Verification items for this drawing (mm, ordinates from the low corner). A direction names the side the tool comes from. Give positions to 0.01 mm unless a question says otherwise; leave off trailing zeros. Write each loop counter-clockwise with the first axis right and the second up, starting at its lowest first coordinate (ties: lowest second). Pieces come first, ordered by that corner, then holes. Notation, with made-up numbers: (-5.75, -5) -> (30.25, -5) arc R15 cw to (30.25, 4) -> close; hole circle Ø9 at (82.5, 22.25). An arc over 180 degrees is marked (long way). Use one line per item in the form item = value. Start each with the question number.
(1) Set-up check for the marked faces 4, 5 and 6: record each of +Z, -Z, +X, -X, +Y, -Y from which the full face is reachable in a straight line by a thin tool's end or side.
(2) Section check B-B, the plane z = 7. Record the cut outline in (x, y).
(3) Release check for a two-part mould opening along Y. For the marked faces 1, 2 and 3 record: pulls with the +Y half, pulls with the -Y half, needs draft (parallel to the pull), parting line crosses it, or undercut.
(4) Depth check by flat-ended pin: pin 1 Ø6 at (x, z) = (14.5, 14.5) entering from -Y; pin 2 Ø4 at (x, y) = (2.5, 229) entering from +Z; pin 3 Ø16.5 at (y, z) = (98.5, 48) entering from -X; pin 4 Ø8 at (x, y) = (36.5, 191.5) entering from -Z. Enter the tip coordinate at first touch or a pass-through.
(5) Section check A-A, the plane x = 55. Record the cut outline in (y, z).
(6) Section check D-D, the plane x = 9. Record the cut outline in (y, z), plus the area to 3 significant figures.
(7) Scan lines: L1, parallel to Y at x = 70, z = 48; L2, parallel to X at y = 227.5, z = 51; L3, parallel to Y at x = 8, z = 6. Record each from-to range of solid material in increasing order.
(8) Section check C-C, the plane y = 227.5. Record the cut outline in (x, z).
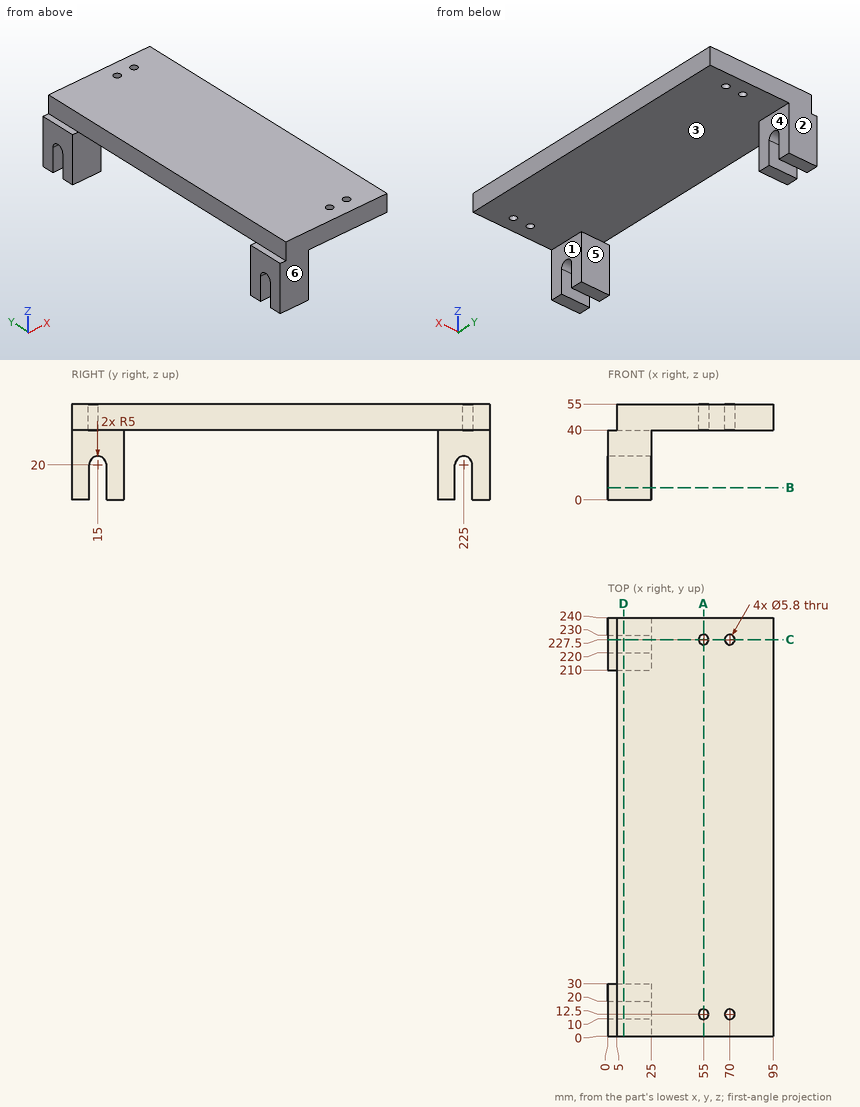
Completed:
q1.face_4 = -Z, +X, +Y, -Y
q1.face_5 = -Z, +X, -X
q1.face_6 = +Z, -Z, +X, -X, -Y
q2.outline = (0, 0) -> (25, 0) -> (25, 10) -> (0, 10) -> close; (0, 20) -> (25, 20) -> (25, 30) -> (0, 30) -> close; (0, 210) -> (25, 210) -> (25, 220) -> (0, 220) -> close; (0, 230) -> (25, 230) -> (25, 240) -> (0, 240) -> close
q3.face_1 = needs draft
q3.face_2 = pulls with the +Y half
q3.face_3 = undercut
q4.pin_1 = 0
q4.pin_2 = 40
q4.pin_3 = 5
q4.pin_4 = 40
q5.outline = (0, 40) -> (9.6, 40) -> (9.6, 55) -> (0, 55) -> close; (15.4, 40) -> (224.6, 40) -> (224.6, 55) -> (15.4, 55) -> close; (230.4, 40) -> (240, 40) -> (240, 55) -> (230.4, 55) -> close
q6.outline = (0, 0) -> (10, 0) -> (10, 20) arc R5 cw to (20, 20) -> (20, 0) -> (30, 0) -> (30, 40) -> (210, 40) -> (210, 0) -> (220, 0) -> (220, 20) arc R5 cw to (230, 20) -> (230, 0) -> (240, 0) -> (240, 55) -> (0, 55) -> close
q6.area = 5,520 mm²
q7.L1 = 0 to 9.6, 15.4 to 224.6, 230.4 to 240
q7.L2 = 5 to 52.1, 57.9 to 67.1, 72.9 to 95
q7.L3 = 0 to 10, 20 to 30, 210 to 220, 230 to 240
q8.outline = (0, 24.33) -> (25, 24.33) -> (25, 40) -> (52.1, 40) -> (52.1, 55) -> (5, 55) -> (5, 40) -> (0, 40) -> close; (57.9, 40) -> (67.1, 40) -> (67.1, 55) -> (57.9, 55) -> close; (72.9, 40) -> (95, 40) -> (95, 55) -> (72.9, 55) -> close
